Source: CAD feature listing. Evaluate the final solid. Frame: model axes, mm. Face numbers are marked on the shaded views. Coordinates: 2 decimals unless noted, no trailing zeros. Loops run counter-clockwise (first coordinate to the right, second up) from the corner with the lowest first, then second, coordinate; pieces in that order, holes last. Notation, with made-up numbers: (87, 48.5) -> (96, 48.5) arc R26 ccw to (96, 71.5) -> close; hole circle Ø10 at (81, 8.5). An arc over 180 degrees is marked (long way). Answer as a JSON object with one key per item and string values. Group by question number.
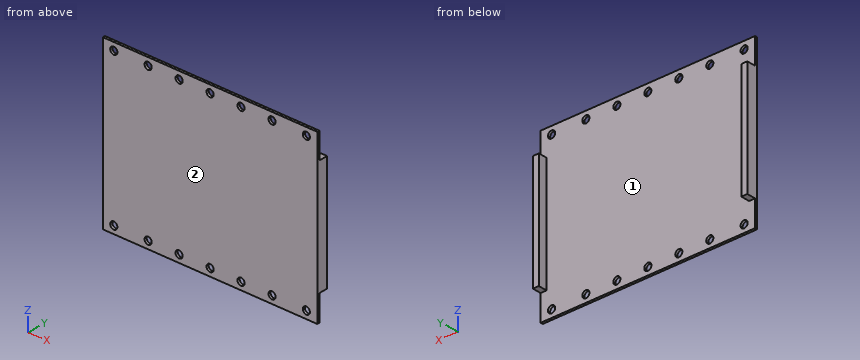
from build123d import *

# Parameters (mm, degrees)
SKETCH_1_W                 = 90
SKETCH_1_H                 = 70
SKETCH_1_R                 = 1.5
EXTRUDE_1_DEPTH            = 1
SKETCH_2_W                 = 2.5
SKETCH_2_H                 = 48.34
EXTRUDE_2_DEPTH            = 3.7
SKETCH_4_R                 = 1.5
CUT_EXTRUDE_1_DEPTH        = 10
PATTERN_LINEAR_1_COUNT     = 3
PATTERN_LINEAR_1_PITCH     = 13
PATTERN_LINEAR_1_COL_COUNT = 3
PATTERN_LINEAR_1_COL_PITCH = 13
MIRROR_2_COPY_1_SKETCH_R   = 1.5
MIRROR_2_COPY_1_DEPTH      = 10
MIRROR_2_COPY_2_SKETCH_R   = 1.5
MIRROR_2_COPY_2_DEPTH      = 10
MIRROR_2_COPY_3_SKETCH_R   = 1.5
MIRROR_2_COPY_3_DEPTH      = 10
MIRROR_2_COPY_4_SKETCH_R   = 1.5
MIRROR_2_COPY_4_DEPTH      = 10


with BuildPart() as part:
    # 草图1 → 凸台-拉伸1 (new body)
    with BuildSketch(Plane(origin=(0, 0, 0), x_dir=(1, 0, 0), z_dir=(0, 1, 0))):
        Rectangle(SKETCH_1_W, SKETCH_1_H)
        with Locations(Location((40.4, -31.85, 0), (0, 0, 270))):
            Circle(SKETCH_1_R, mode=Mode.SUBTRACT)
        with Locations(Location((-40.4, -31.85, 0), (0, 0, 90))):
            Circle(SKETCH_1_R, mode=Mode.SUBTRACT)
        with Locations(Location((40.4, 31.85, 0), (0, 0, 90))):
            Circle(SKETCH_1_R, mode=Mode.SUBTRACT)
        with Locations(Location((-40.4, 31.85, 0), (0, 0, 270))):
            Circle(SKETCH_1_R, mode=Mode.SUBTRACT)
    extrude(amount=EXTRUDE_1_DEPTH)

    # 草图2 → 凸台-拉伸2 (add)
    with BuildSketch(Plane(origin=(0, 1, 0), x_dir=(1, 0, 0), z_dir=(0, 1, 0))):
        with Locations((43.75, 0)):
            Rectangle(SKETCH_2_W, SKETCH_2_H)
    extrude_2 = extrude(amount=EXTRUDE_2_DEPTH)

    # 镜向1: 凸台-拉伸2 across plane
    add(extrude_2.mirror(Plane(origin=(0, 0, 0), x_dir=(0, 0, 1), z_dir=(1, 0, 0))))

    # 草图4 → 切除-拉伸1 (cut)
    with BuildSketch(Plane.XZ):
        with Locations(Location((0, 31.85, 0), (0, 0, 270))):
            Circle(SKETCH_4_R)
    cut_extrude_1 = extrude(amount=-CUT_EXTRUDE_1_DEPTH, mode=Mode.SUBTRACT)

    # 阵列(线性)1: 切除-拉伸1 ×3
    with Locations(*[(-i * PATTERN_LINEAR_1_PITCH, 0, 0) for i in range(1, PATTERN_LINEAR_1_COUNT)]):
        add(cut_extrude_1, mode=Mode.SUBTRACT)

    # 阵列(线性)1 col: 切除-拉伸1 ×3
    with Locations(*[(i * PATTERN_LINEAR_1_COL_PITCH, 0, 0) for i in range(1, PATTERN_LINEAR_1_COL_COUNT)]):
        add(cut_extrude_1, mode=Mode.SUBTRACT)

    # 镜向2: 切除-拉伸1 across plane
    add(cut_extrude_1.mirror(Plane.XY), mode=Mode.SUBTRACT)

    # 镜向2 copy 1 sketch → 镜向2 copy 1 (cut)
    with BuildSketch(Plane(origin=(-13, 0, 0), x_dir=(1, 0, 0), z_dir=(0, -1, 0))):
        with Locations((0, -31.85)):
            Circle(MIRROR_2_COPY_1_SKETCH_R)
    extrude(amount=-MIRROR_2_COPY_1_DEPTH, mode=Mode.SUBTRACT)

    # 镜向2 copy 2 sketch → 镜向2 copy 2 (cut)
    with BuildSketch(Plane(origin=(-26, 0, 0), x_dir=(1, 0, 0), z_dir=(0, -1, 0))):
        with Locations((0, -31.85)):
            Circle(MIRROR_2_COPY_2_SKETCH_R)
    extrude(amount=-MIRROR_2_COPY_2_DEPTH, mode=Mode.SUBTRACT)

    # 镜向2 copy 3 sketch → 镜向2 copy 3 (cut)
    with BuildSketch(Plane(origin=(13, 0, 0), x_dir=(1, 0, 0), z_dir=(0, -1, 0))):
        with Locations((0, -31.85)):
            Circle(MIRROR_2_COPY_3_SKETCH_R)
    extrude(amount=-MIRROR_2_COPY_3_DEPTH, mode=Mode.SUBTRACT)

    # 镜向2 copy 4 sketch → 镜向2 copy 4 (cut)
    with BuildSketch(Plane(origin=(26, 0, 0), x_dir=(1, 0, 0), z_dir=(0, -1, 0))):
        with Locations((0, -31.85)):
            Circle(MIRROR_2_COPY_4_SKETCH_R)
    extrude(amount=-MIRROR_2_COPY_4_DEPTH, mode=Mode.SUBTRACT)


solid = part.part
1. Mould query, pull axis X, two halves, no side actions, for the marked faces 1 and 2. Classes: pulls with the +X half, pulls with the -X half, needs draft (parallel to the pull), parting line crosses it, or undercut.
2. Section query C-C on y = 2.35. Return loops of the section in (x, z), then the cut area to 3 significant figures.
3. Section query A-A on z = -31.85. State how many separate pieces and enclosed holes the cut face has, then the cut area to 3 significant figures.
4. Pin query (flat end, axial travel): pin 1 Ø2 at (x, y) = (-43.5, 2.5) entering from -Z; pin 2 Ø4 at (x, z) = (26, -31.85) entering from +Y. Return the tip coordinate at first contact, or that it passes through.
5. Section query D-D on z = -5. Return loops of the section in (x, y), then the cut area to 4 significant figures.
6. Ray query, L1, parallel to X at y = 2.55, z = -11; L2, parallel to Y at x = 28, z = -8. Return the intervals inside material, ascending.
7. Section query B-B on x = -13. Return loops of the section in (y, z), then the cut area to 3 significant figures.
Solved:
{
 "1": {"face 1": "undercut", "face 2": "needs draft"},
 "2": {"outline": "(-45, -24.17) -> (-42.5, -24.17) -> (-42.5, 24.17) -> (-45, 24.17) -> close; (42.5, -24.17) -> (45, -24.17) -> (45, 24.17) -> (42.5, 24.17) -> close", "area": "242 mm^2"},
 "3": {"separate pieces": "8", "enclosed holes": "0", "area": "69.0 mm^2"},
 "4": {"pin 1": "z = -24.17", "pin 2": "y = 1"},
 "5": {"outline": "(-45, 0) -> (45, 0) -> (45, 4.7) -> (42.5, 4.7) -> (42.5, 1) -> (-42.5, 1) -> (-42.5, 4.7) -> (-45, 4.7) -> close", "area": "108.5 mm^2"},
 "6": {"L1": "-45 to -42.5, 42.5 to 45", "L2": "0 to 1"},
 "7": {"outline": "(0, -35) -> (1, -35) -> (1, -33.35) -> (0, -33.35) -> close; (0, -30.35) -> (1, -30.35) -> (1, 30.35) -> (0, 30.35) -> close; (0, 33.35) -> (1, 33.35) -> (1, 35) -> (0, 35) -> close", "area": "64.0 mm^2"}
}
